```python
from build123d import *

# Parameters (mm, degrees)
F0_W     = 50.8
F0_H     = 50.8
F1_DEPTH = 50.8
F2_R     = 13.395396
F3_DEPTH = 61.722
F4_W     = 25.4
F4_H     = 25.4
F5_DEPTH = 12.7
F6_R     = 12.7
F7_DEPTH = 12.7


with BuildPart() as f1:
    # F0 (on Front) → F1 (new body)
    with BuildSketch(Plane.XZ):
        with Locations((-25.4, 25.4)):
            Rectangle(F0_W, F0_H)
    extrude(amount=F1_DEPTH)

    # F2 (on face) → F3 (cut)
    with BuildSketch(Plane.XZ.offset(50.8)):
        with Locations((-26.095396, 26.924606)):
            Circle(F2_R)
    extrude(amount=-F3_DEPTH, mode=Mode.SUBTRACT)

    # F4 (on face) → F5 (join)
    with BuildSketch(Plane(origin=(-50.8, 0, 0), x_dir=(0, -1, 0), z_dir=(-1, 0, 0))):
        with Locations((25.4, 25.4)):
            Rectangle(F4_W, F4_H)
    extrude(amount=F5_DEPTH)

    # F6 (on face) → F7 (join)
    with BuildSketch(Plane(origin=(0, 0, 0), x_dir=(1, 0, 0), z_dir=(0, 0, -1))):
        with Locations((-25.4, 25.4)):
            Circle(F6_R)
    extrude(amount=F7_DEPTH)


solid = f1.part
```
Verification items for the finished model (mm, model axes). A direction names the side the tool comes from. Give positions to 0.01 mm unless a question says otherwise; leave off trailing zeros. Write each loop counter-clockwise with the first axis right and the second up, starting at its lowest first coordinate (ties: lowest second). Pieces come first, ordered by that corner, then holes. Notation, with made-up numbers: (-2.75, 65) - (1.25, 65) arc R28 cw to (1.25, 89) - close; hole circle Ø11 at (-39, 29.5). An arc over 180 degrees is marked (long way). Put each result on its own line as item: value.
Q1. Section check A-A on z = 19.5. Record the cut outline in (x, y).
Result:
outline: (-63.5, -38.1) - (-50.8, -38.1) - (-50.8, -50.8) - (-37.24, -50.8) - (-37.24, 0) - (-50.8, 0) - (-50.8, -12.7) - (-63.5, -12.7) - close; (-14.95, -50.8) - (0, -50.8) - (0, 0) - (-14.95, 0) - close
Q2. Scan lines: probe 1 along X at (y, z) = (-25, 27); probe 2 along X at (y, z) = (-6.5, 26.5); probe 3 along Z at (x, y) = (-48.5, -7). Record each from-to range of solid material in increasing order. Write a range as from..to.
Result:
probe 1: -63.5..-39.49, -12.7..0
probe 2: -50.8..-39.48, -12.71..0
probe 3: 0..50.8
Q3. Section check B-B on x = -36. Record the cut outline in (y, z) (3 decimals).
Result:
outline: (-50.8, 0) - (-32.395, 0) - (-32.395, -12.7) - (-18.405, -12.7) - (-18.405, 0) - (0, 0) - (0, 17.906) - (-50.8, 17.906) - close; (-50.8, 35.943) - (0, 35.943) - (0, 50.8) - (-50.8, 50.8) - close
Q4. Depth check by flat-ended pin: P1, Ø3, axis at x = -52.5, y = -38.5, coming from the -Z side; P2, Ø6.5, axis at x = -60, y = -27.5, coming from the +Z side; P3, Ø3, axis at x = -17, z = 32, coming from the +Y side; P4, Ø10, axis at x = -57, z = 29, coming from the +Y side. Enter the tip coordinate at first touch or a pass-through.
Result:
P1: z = 12.7
P2: z = 38.1
P3: through
P4: y = -12.7
Q5. Mould release check, pull along X, two halves, no side actions. Record for faces 1 (the face through (-31.4, -13.8, 0)), 2 (the face through (-28.999, -25.756, 13.848)), 3 (the face through (-18.573, -36.109, -6.261)): released by +X, released by -X, zero draft, split by the parting line, or undercut.
Result:
face 1: zero draft
face 2: undercut
face 3: split by the parting line
Q6. Section check C-C on y = -25.4. Record the cut outline in (x, z), and give its area (3 significant figures).
Result:
outline: (-63.5, 12.7) - (-50.8, 12.7) - (-50.8, 0) - (-38.1, 0) - (-38.1, -12.7) - (-12.7, -12.7) - (-12.7, 0) - (0, 0) - (0, 50.8) - (-50.8, 50.8) - (-50.8, 38.1) - (-63.5, 38.1) - close; hole circle Ø26.79 at (-26.1, 26.92)
area: 2,660 mm2
Q7. Set-up check for faces 4 (the face through (-57, -12.7, 25)), 5 (the face through (-57, -25, 12.7)), 6 (the face through (-57, -25, 38.1)), 7 (the face through (-57, -38.1, 25)): record each of +Z, -Z, +X, -X, +Y, -Y from which the full face is reachable in a straight line by a thin tool's end or side.
Result:
face 4: +Z, -Z, -X, +Y
face 5: -Z, -X, +Y, -Y
face 6: +Z, -X, +Y, -Y
face 7: +Z, -Z, -X, -Y
Q8. Section check D-D on z = 11.5. Record the cut outline in (x, y).
Result:
outline: (-50.8, -50.8) - (0, -50.8) - (0, 0) - (-50.8, 0) - close
